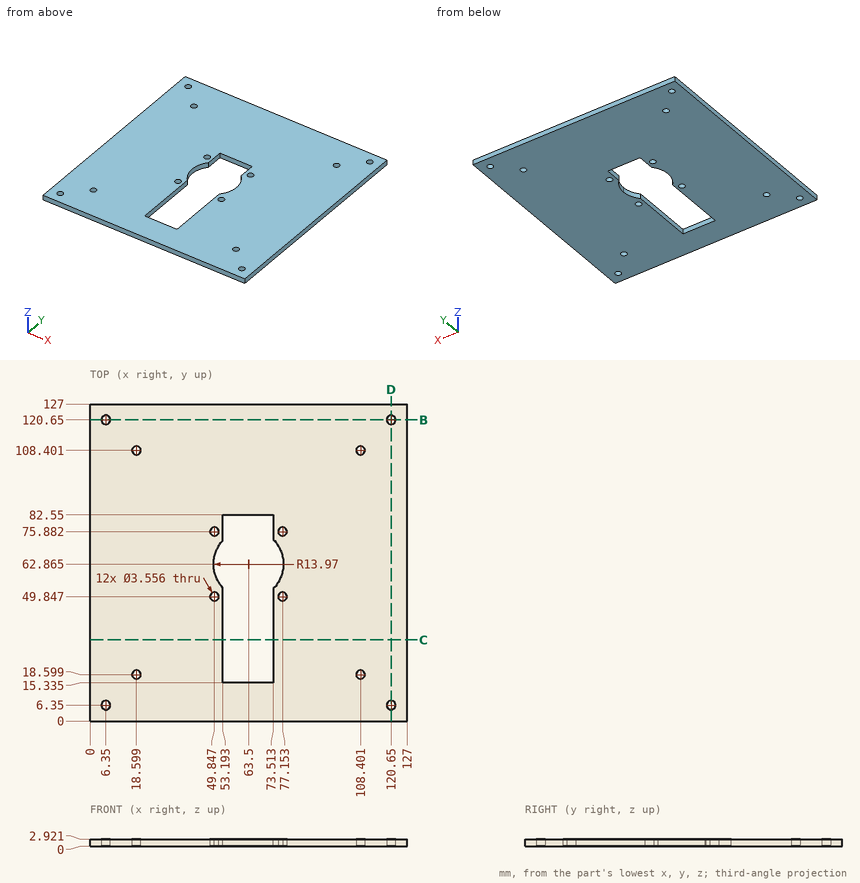
Input: dimensioned drawing with shaded views. Units: mm. Origin: part minimum x, y, z. Coordinates: 2 decimals unless noted, no trailing zeros. Loops run counter-clockwise (first coordinate to the right, second up) from the corner with the lowest first, then second, coordinate; pieces in that order, holes last. Notation, with made-up numbers: M 70,-0.75 L 120,-0.75 A24 ccw 120,25.25 Z; hole C 66.25,-19 d1. An arc over 180 degrees is marked long. One line per item, written item: value. Start each with the question number.
1) Cut plane C-C (y = 32.5). Return loops of the section in (x, z).
2) Cut plane B-B (y = 120.65). Return loops of the section in (x, z).
3) Material intervals for L1, parallel to X at y = 120.65, z = 1.4; L2, parallel to X at y = 42.5, z = 2.75, sorted ascending. Write a range as from..to.
Evaluation:
1. outline: M 0,0 L 53.19,0 L 53.19,2.92 L 0,2.92 Z; M 73.51,0 L 127,0 L 127,2.92 L 73.51,2.92 Z
2. outline: M 0,0 L 4.57,0 L 4.57,2.92 L 0,2.92 Z; M 8.13,0 L 118.87,0 L 118.87,2.92 L 8.13,2.92 Z; M 122.43,0 L 127,0 L 127,2.92 L 122.43,2.92 Z
3. L1: 0..4.57, 8.13..118.87, 122.43..127
3. L2: 0..53.19, 73.51..127
